Autodesk Inventor part; units mm, degrees
ref_plane "YZ Plane" through (0, 0, 0) normal (1, 0, 0) x (0, 1, 0)
ref_plane "XZ Plane" through (0, 0, 0) normal (0, 1, 0) x (-1, 0, 0)
ref_plane "XY Plane" through (0, 0, 0) normal (0, 0, 1) x (1, 0, 0)
sketch "Sketch1" plane through (0, 0, 0) normal (0, 1, 0) x (-1, 0, 0)
  line L0 (0, 0) -> (41.148, 0)
  line L1 (41.148, 0) -> (41.148, -20.32)
  line L2 (41.148, -20.32) -> (0, -20.32)
  line L3 (0, -20.32) -> (0, 0)
  circle A0 centre (45.212, -15.24) radius 2.0193
  circle A1 centre (-4.064, -15.24) radius 2.0193
  circle A2 centre (45.212, -5.08) radius 2.0193
  circle A3 centre (-4.064, -5.08) radius 2.0193
  line L4 (41.148, -9.652) -> (49.276, -9.652)
  line L5 (41.148, -10.668) -> (49.276, -10.668)
  line L6 (-8.128, -9.652) -> (0, -9.652)
  line L7 (-8.128, -10.668) -> (0, -10.668)
  line L8 (-8.128, 3.81) -> (49.276, 3.81)
  line L9 (49.276, 3.81) -> (49.276, -24.13)
  line L10 (49.276, -24.13) -> (-8.128, -24.13)
  line L11 (-8.128, -24.13) -> (-8.128, 3.81)
  line L12 (-6.155, -5.4575) -> (-6.0508, -5.4409)
  line L13 (-6.155, -5.4575) -> (-6.0508, -5.4409)
  line L14 (20.574, -20.32) -> (20.574, 0)
  circle A4 centre (10.668, -10.16) radius 6.604
  circle A5 centre (-4.318, 9.4045) radius 2.0193
  line L15 (-8.128, 13.2145) -> (34.4551, 13.2145)
  circle A6 centre (30.6451, 9.4045) radius 2.0193
  circle A7 centre (30.6451, -27.1845) radius 2.0193
  line L16 (10.668, -30.9945) -> (34.4551, -30.9945)
  line L17 (-8.128, -30.9945) -> (34.4551, -30.9945)
  circle A8 centre (-5.588, -28.4545) radius 2.0193
  line L18 (34.4551, -30.9945) -> (-8.128, -30.9945)
  line L19 (-8.128, -30.9945) -> (-8.128, 13.2145)
  line L20 (-8.128, 13.2145) -> (34.4551, 13.2145)
  line L21 (34.4551, -24.13) -> (34.4551, -30.9945)
  line L22 (34.4551, 13.2145) -> (34.4551, 3.81)
  circle A9 centre (30.6451, 9.4045) radius 2.286
  circle A10 centre (-4.318, 9.4045) radius 2.286
  circle A11 centre (-5.588, -28.4545) radius 2.286
  circle A12 centre (30.6451, -27.1845) radius 2.286
  point P0 (20.574, -10.16)
  point P1 (-8.128, -24.13)
  point P2 (-8.128, 3.81)
  dimension "d0" = 41.148
  dimension "d1" = 20.32
  dimension "d4" = 4.0386
  dimension "d5" = 4.0386
  dimension "d18" = 4.064
  dimension "d19" = 4.064
  dimension "d52" = 8.128
  dimension "d53" = 8.128
  dimension "d54" = 3.81
  dimension "d55" = 3.81
  dimension "d59" = 9.906
  dimension "d60" = 13.208
  dimension "d79" = 4.0386
  dimension "d80" = 4.0386
  dimension "d81" = 4.0386
  dimension "d82" = 4.0386
  dimension "d84" = 3.81
  dimension "d91" = 4.572
  dimension "d92" = 4.572
  dimension "d93" = 4.572
  dimension "d94" = 4.572
extrude "Extrusion10" add sketch "Sketch1" along normal blind 11.811 contours L3 L6 L11 L8 L9 L4 L1 L0 | L0 L14 L2 L3 | L0 L1 L2 L14 | L3 L7 L11 L6 | L2 L1 L5 L9 L10 L11 L7 L3 | L4 L9 L5 L1
extrude "Extrusion11" cut sketch "Sketch1" along normal blind 10.16 contours L0 L14 L2 L3 | L0 L1 L2 L14
extrude "Extrusion12" cut sketch "Sketch1" along normal blind 2.032 contours L3 L7 L11 L6 | L4 L9 L5 L1
extrude "Extrusion13" add sketch "Sketch1" along normal up to surface (11.811 mm away) contours L19 L15 L22 L8 | L10 L21 L16 L17 L19 | A8 | A11
properties part number "Servo Mount"
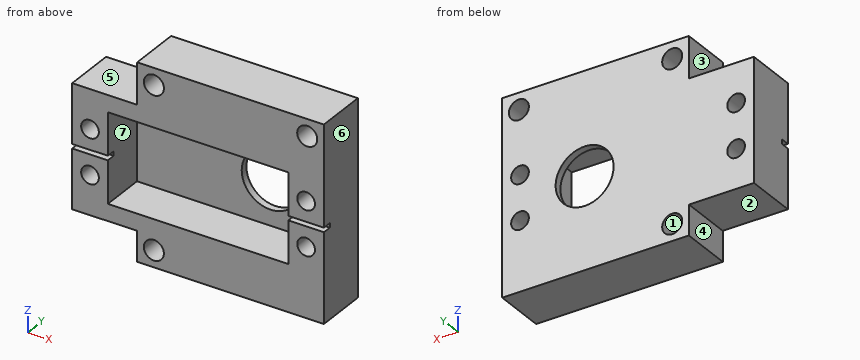
Can you work these out from the model? Positions are in its coordinate system, mm. Face numbers are marked on the shaded views. A direction names the side the tool comes from. Give positions to 0.01 mm unless a question says otherwise; leave off trailing zeros. Order: outer loops, then holes, each group sorted by start corner. A loop starts at its lowest first (then second) coordinate and runs counter-clockwise, first axis right, second up. Notation, with made-up numbers: M 9,38.25 L 47,38.25 A31 ccw 47,69.25 Z; hole C 23.25,-12.75 d4. An arc over 180 degrees is marked long. One line per item, written item: value.
Item 1: If we section it at C-C on x = -38: Write out the boundary of the cut face in (y, z), and give its area (3 significant figures).
Verdict:
outline: M 0,-24.13 L 11.81,-24.13 L 11.81,3.81 L 0,3.81 L 0,0 L 10.16,0 L 10.16,-20.32 L 0,-20.32 Z
area: 124 mm2
Item 2: If we mould it in two halves opening along X, with no side actions, what happens to the marked faces 1, 2 and 3? For each: pulls with the +X half, pulls with the -X half, needs draft (parallel to the pull), parting line crosses it, or undercut.
Verdict:
face 1: undercut
face 2: needs draft
face 3: pulls with the -X half
Item 3: Please list where these lines run through material, in increasing order: line 1 (X direction, y = 1.75, z = 9.5); line 2 (Z direction, x = -23.5, y = 7); line 3 (X direction, y = 2, z = -27).
Verdict:
line 1: -34.46 to -32.93, -28.36 to 2.03, 6.6 to 8.13
line 2: -30.99 to -20.32, 0 to 13.21
line 3: -34.46 to -32.92, -28.37 to 8.13
Item 4: If we section it at A-A on z = -5.08: Write out the boundary of the cut face in (x, y), and give its area (3 significant figures).
Verdict:
outline: M -49.28,0 L -47.23,0 L -47.23,11.81 L -49.28,11.81 Z; M -43.19,0 L -41.15,0 L -41.15,10.16 L -14.89,10.16 L -14.89,11.81 L -43.19,11.81 Z; M -6.45,10.16 L 0,10.16 L 0,0 L 2.04,0 L 2.04,11.81 L -6.45,11.81 Z; M 6.08,0 L 8.13,0 L 8.13,11.81 L 6.08,11.81 Z
area: 151 mm2
Item 5: For the marked faces 4, 5, 6 and 7, which set-ups out of +Z, -Z, +X, -X, +Y, -Y let a thin tool reach every point of the face, with its end or its side?
Verdict:
face 4: -Z, -X, +Y, -Y
face 5: +Z, -X, +Y, -Y
face 6: +Z, -Z, +X, +Y, -Y
face 7: -Y
Item 6: If we section it at D-D on z = 8: Write out the boundary of the cut face in (x, y), and give its area (3 significant figures).
Verdict:
outline: M -34.46,0 L -32.45,0 L -32.45,11.81 L -34.46,11.81 Z; M -28.84,0 L 2.51,0 L 2.51,11.81 L -28.84,11.81 Z; M 6.12,0 L 8.13,0 L 8.13,11.81 L 6.12,11.81 Z
area: 418 mm2
Item 7: If we section it at B-B on x = 3: Write out the boundary of the cut face in (y, z), and give its area (3 significant figures).
Verdict:
outline: M 0,-30.99 L 11.81,-30.99 L 11.81,-16.96 L 0,-16.96 Z; M 0,-13.52 L 11.81,-13.52 L 11.81,-6.8 L 0,-6.8 L 0,-9.65 L 2.03,-9.65 L 2.03,-10.67 L 0,-10.67 Z; M 0,-3.36 L 11.81,-3.36 L 11.81,7.54 L 0,7.54 Z; M 0,11.27 L 11.81,11.27 L 11.81,13.21 L 0,13.21 Z
area: 395 mm2
Item 8: For pin 1 (3.5 mm diameter, centred on x = -42, y = 4.5, fed in from -Z); pin 2 (2.5 mm diameter, centred on x = -30.65, z = -27.18, fed in from -Y); pin 3 (1 mm diameter, centred on x = -37.5, z = -2, fed in from -Y); pin 4 (2 mm diameter, centred on x = -39, y = 5, fed in from +Z), each with a flat end and sliding along its axis, tell me the tip position at first contact or that it passes through.
Verdict:
pin 1: z = -24.13
pin 2: through
pin 3: y = 10.16
pin 4: z = 3.81
